Print and shaded views of the part. All mm, measured from the part's lowest x, y and z. A direction names the side the tool comes from. Round coordinates to 2 decimals unless told otherwise and drop trailing zeros. Use one line per item in the form item = value.
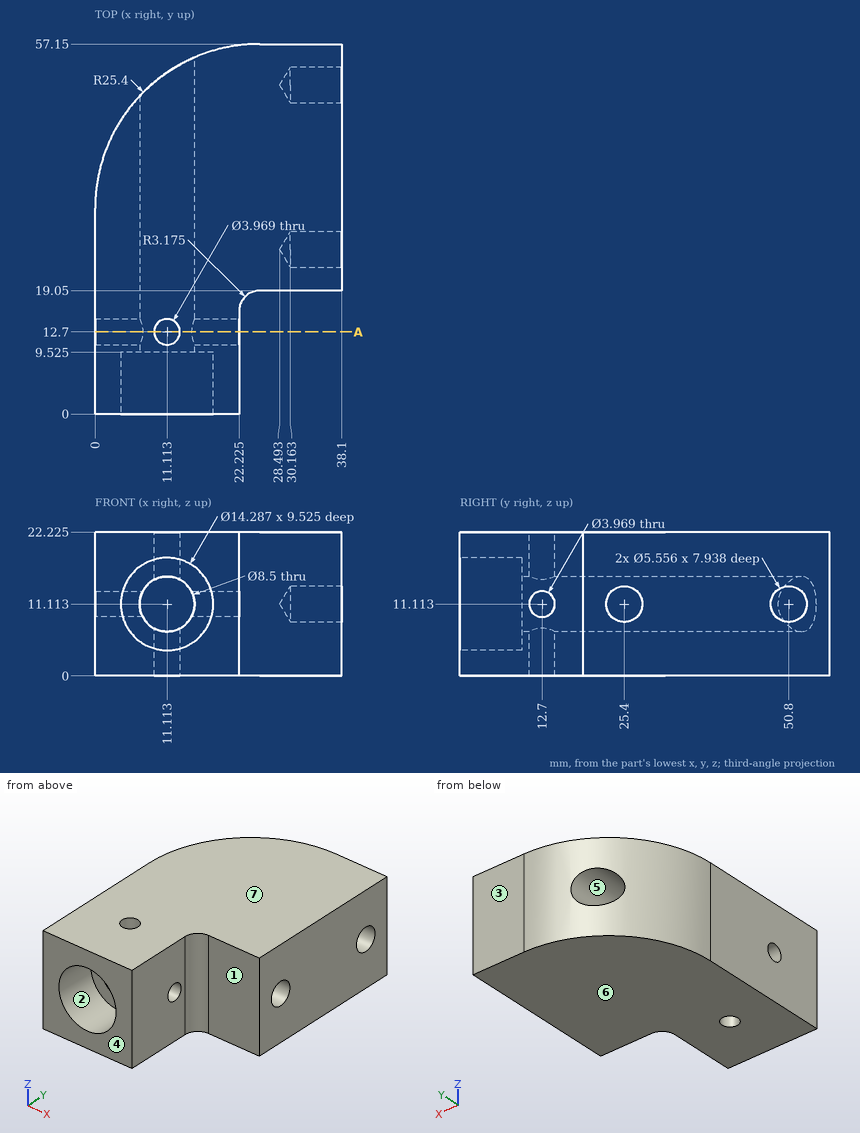
1) Flat gauge pins, fed straight in: pin 1 (4.5 mm diameter, centred on x = 8.5, z = 9.5, fed in from -Y) (1 decimal); pin 2 (4.5 mm diameter, centred on y = 12.7, z = 11.11, fed in from +X) (1 decimal); pin 3 (6.5 mm diameter, centred on x = 31, z = 7.5, fed in from -Y). Where does each tip first touch, or does it go through?
Report:
pin_1 = 9.5
pin_2 = 22.2
pin_3 = 19.05
2) Drill centre lines: probe 1 along X at (y, z) = (12.7, 3.5) (1 decimal); probe 2 along Y at (x, z) = (27.5, 11.75); probe 3 along Z at (x, y) = (34.25, 50.8) (1 decimal). Where is each one in solid material? Low to high.
Report:
probe_1 = 0 to 9.1, 13.1 to 22.2
probe_2 = 19.05 to 57.15
probe_3 = 0 to 8.3, 13.9 to 22.2
3) Slice it at A-A (y = 12.7). State how many separate pieces and enclosed holes the cut face has, plus the area to 3 significant figures.
Report:
separate_pieces = 4
enclosed_holes = 0
area = 326 mm^2
4) Tool access for the marked faces 1, 2 and 3: list every direction of +Z, -Z, +X, -X, +Y, -Y with a clear straight run to the whole face (end or side of a thin tool).
Report:
face_1 = +Z, -Z, +X, -Y
face_2 = -Y
face_3 = +Z, -Z, +X, -X, +Y
5) Two-plate mould, pull along Z, no slides. Class the marked faces 4, 5, 6 and 7: +Z half, -Z half, draft (parallel to the pull), parting line (faces both ways), or undercut.
Report:
face_4 = draft
face_5 = undercut
face_6 = -Z half
face_7 = +Z half
